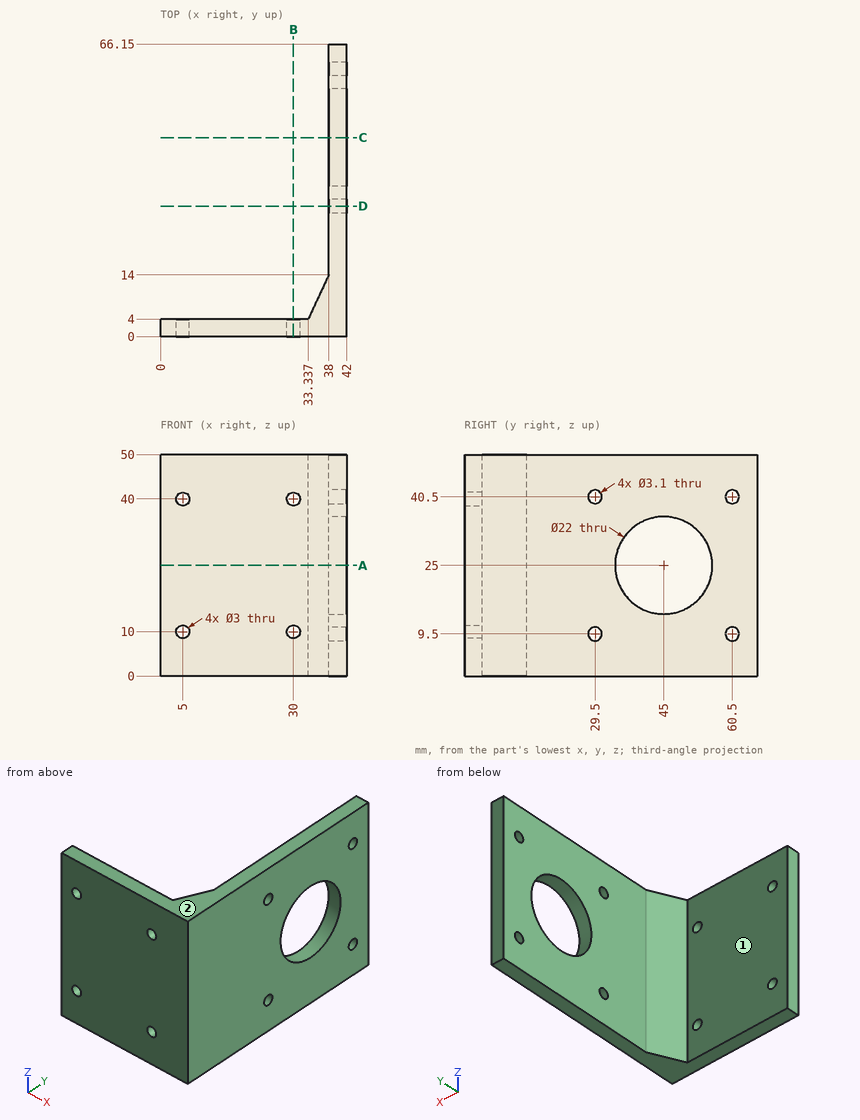
Check sheet for the drawn part. Datum: minimum x, y, z corner. Units: mm. A direction names the side the tool comes from. Give positions to 0.01 mm unless a question says otherwise; leave off trailing zeros. Order: outer loops, then holes, each group sorted by start corner. A loop starts at its lowest first (then second) coordinate and runs counter-clockwise, first axis right, second up. Notation, with made-up numbers: (-36, 85) - (-29, 85) arc R24 cw to (-29, 117) - close; hole circle Ø3 at (61.5, 88). An arc over 180 degrees is marked (long way). Answer as a JSON object with one key per item and string values.
(1) Material ranges on line 1 (X direction, y = 2, z = 10); line 2 (Y direction, x = 41.25, z = 40.5); line 3 (Z direction, x = 5, y = 3.05), recorded low to high.
Report:
{"line 1": "0 to 3.5, 6.5 to 28.5, 31.5 to 42", "line 2": "0 to 27.95, 31.05 to 58.95, 62.05 to 66.15", "line 3": "0 to 8.5, 11.5 to 38.5, 41.5 to 50"}
(2) Cross-section at C-C (y = 45). Record the cut outline in (x, z), then the cut area to 3 significant figures.
Report:
{"outline": "(38, 0) - (42, 0) - (42, 14) - (38, 14) - close; (38, 36) - (42, 36) - (42, 50) - (38, 50) - close", "area": "112 mm^2"}
(3) Cross-section at B-B (x = 30). Record the cut outline in (y, z).
Report:
{"outline": "(0, 0) - (4, 0) - (4, 8.5) - (0, 8.5) - close; (0, 11.5) - (4, 11.5) - (4, 38.5) - (0, 38.5) - close; (0, 41.5) - (4, 41.5) - (4, 50) - (0, 50) - close"}
(4) Depth check by flat-ended pin: pin 1 Ø5 at (y, z) = (60.5, 40.5) entering from -X; pin 2 Ø1 at (x, z) = (20.5, 10.5) entering from +Y; pin 3 Ø2 at (x, z) = (33, 34) entering from +Y. Enter the tip coordinate at first touch or a pass-through.
Report:
{"pin 1": "x = 38", "pin 2": "y = 4", "pin 3": "y = 5.42"}
(5) Cross-section at A-A (z = 25). Record the cut outline in (x, y), then the cut area to 3 significant figures.
Report:
{"outline": "(0, 0) - (42, 0) - (42, 34) - (38, 34) - (38, 14) - (33.34, 4) - (0, 4) - close; (38, 56) - (42, 56) - (42, 66.15) - (38, 66.15) - close", "area": "352 mm^2"}
(6) Tool access check on the marked faces 1 and 2. Record the directions out of +Z, -Z, +X, -X, +Y, -Y that give a thin tool (end or side, any length) a straight path to the whole face; none if there is none.
Report:
{"face 1": "+Z, -Z, -X, +Y", "face 2": "+Z, +X, -X, +Y, -Y"}
(7) Cross-section at D-D (y = 29.5). Record the cut outline in (x, z), then the cut area to 3 significant figures.
Report:
{"outline": "(38, 0) - (42, 0) - (42, 7.95) - (38, 7.95) - close; (38, 11.05) - (42, 11.05) - (42, 38.95) - (38, 38.95) - close; (38, 42.05) - (42, 42.05) - (42, 50) - (38, 50) - close", "area": "175 mm^2"}
